from build123d import *

# Parameters (mm, degrees)
BOSS_EXTRU_1_DEPTH = 50


with BuildPart() as part:
    # Esquisse1 → Boss.-Extru.1 (new body)
    with BuildSketch(Plane(origin=(0, 0, 0), x_dir=(1, 0, 0), z_dir=(0, 1, 0))):
        with BuildLine():
            Line((15.419133563, -15.419133563), (15.419133563, 15.419133563))
            Line((15.419133563, 15.419133563), (-15.419133563, 15.419133563))
            Line((-15.419133563, 15.419133563), (-24.494437672, 15.419133563))
            Line((-24.494437672, 15.419133563), (-193.160150167, -18.138198396))
            Line((-193.160150167, -18.138198396), (-193.160150167, -28.234642357))
            Line((-193.160150167, -28.234642357), (-182.185114876, -28.234642357))
            add(Edge.make_bspline(
                [(-182.185114876, -28.234642357), (-99.136016822, -17.08659502), (-15.419133563, -15.419133563)],
                knots=[0, 0, 0, 1, 1, 1], degree=2))
            Line((-15.419133563, -15.419133563), (-5.487517645, -28.234642357))
            Line((-5.487517645, -28.234642357), (5.487517645, -28.234642357))
            Line((5.487517645, -28.234642357), (15.419133563, -15.419133563))
        make_face()
        Polygon((-10.073577327, 10.1), (-2.373577327, 10.1), (-2.373577327, 3.85), (2.373577327, 3.85), (2.373577327, 10.1), (10.126422673, 10.1), (10.126422673, 2.4), (3.876422673, 2.4), (3.876422673, -2.4), (10.126422673, -2.4), (10.126422673, -10.1), (2.426422673, -10.1), (2.426422673, -3.85), (-2.373577327, -3.85), (-2.373577327, -10.1), (-10.073577327, -10.1), (-10.073577327, -2.4), (-3.823577327, -2.4), (-3.823577327, 2.4), (-10.073577327, 2.4), align=None, mode=Mode.SUBTRACT)
        with BuildLine():
            Line((-23.518772506, 10.515249645), (-188.160150167, -22.241410157))
            Line((-188.160150167, -22.241410157), (-188.160150167, -23.234642357))
            Line((-188.160150167, -23.234642357), (-182.518919813, -23.234642357))
            add(Edge.make_bspline(
                [(-182.518919813, -23.234642357), (-99.352804626, -12.089945504), (-15.518703132, -10.420125071)],
                knots=[0.001988478, 0.001988478, 0.001988478, 1, 1, 1], degree=2))
            Line((-15.518703132, -10.420125071), (-23.518772506, 10.515249645))
        make_face(mode=Mode.SUBTRACT)
    extrude(amount=BOSS_EXTRU_1_DEPTH)


solid = part.part
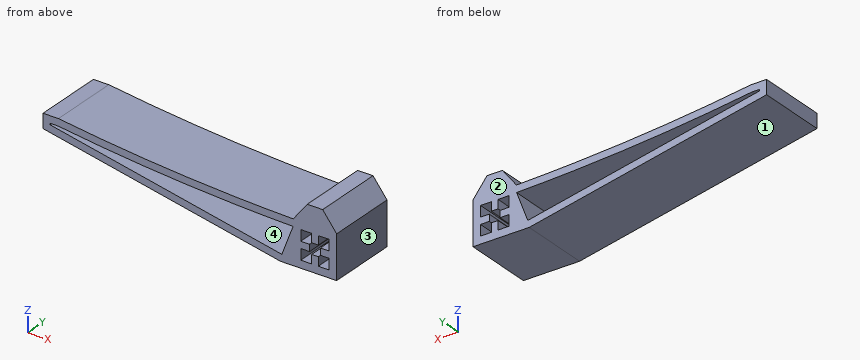
Source: CAD feature listing. Evaluate the final solid. Frame: model axes, mm. Face numbers are marked on the shaded views. Round coordinates to 2 decimals unless told otherwise and drop trailing zeros. Loops run counter-clockwise (first coordinate to the right, second up) from the corner with the lowest first, then second, coordinate; pieces in that order, holes last.
Q1. Section A-A, the plane z = 0. Return loops of the section in (x, y).
Q2. First-contact query: P1, Ø1.1, axis at y = 19, z = 22.5, coming from the +X side; P2, Ø1.7, axis at x = -186, y = 34.5, coming from the -Z side; P3, Ø2, axis at x = -131.5, y = 35.5, coming from the -Z side. Flat tips, straight axial feed; report the tip coordinate or a pass-through.
Q3. Mould query, pull axis X, two halves, no side actions, for the marked faces 1, 2, 3 and 4. Classes: pulls with the +X half, pulls with the -X half, needs draft (parallel to the pull), parting line crosses it, or undercut.
Q4. Section B-B, the plane y = 44.5. State how many separate pieces and enclosed holes the cut face has, plus the area to 3 significant figures.
Q5. Ray query, line 1 (Z direction, x = -33, y = 29); line 2 (Z direction, x = -153, y = 47); line 3 (Z direction, x = -14, y = 20). Return the intervals inside material, ascending.
Solutions:
1. outline: (-101.99, 0) - (-76.37, 0) - (-76.37, 50) - (-101.99, 50) - close; (-19.5, 0) - (-3.82, 0) - (-3.82, 50) - (-19.5, 50) - close; (3.88, 0) - (15.42, 0) - (15.42, 50) - (3.88, 50) - close
2. P1: stops at x = 10.36
2. P2: stops at z = 16.54
2. P3: stops at z = 5.67
3. face 1: pulls with the -X half
3. face 2: needs draft
3. face 3: pulls with the +X half
3. face 4: undercut
4. separate pieces: 1
4. enclosed holes: 2
4. area: 2,810 mm2
5. line 1: z = -13.73 to -8.63, 10.87 to 15.87
5. line 2: z = 10.15 to 15.25, 19.58 to 24.61
5. line 3: z = -15.42 to 17.25
